from build123d import *

# Parameters (mm, degrees)
ESQUISSE1_W                = 98.15
ESQUISSE1_H                = 27.3
BOSS_EXTRU_1_DEPTH         = 2.7
ESQUISSE2_W                = 10
ESQUISSE2_H                = 2.7
BOSS_EXTRU_2_DEPTH         = 2.7
R_P_TITION_LIN_AIRE1_COUNT = 5
R_P_TITION_LIN_AIRE1_PITCH = 20
ESQUISSE3_W                = 2.7
ESQUISSE3_H                = 6.5
BOSS_EXTRU_3_DEPTH         = 2.7
R_P_TITION_LIN_AIRE2_COUNT = 2
R_P_TITION_LIN_AIRE2_PITCH = 13
ENL_V_MAT_EXTRU_1_DEPTH    = 2.7
CONG_1_R                   = 30
ESQUISSE5_W                = 2.7
ESQUISSE5_H                = 9.15
ENL_V_MAT_EXTRU_2_DEPTH    = 2.7


with BuildPart() as part:
    # Esquisse1 → Boss.-Extru.1 (new body)
    with BuildSketch(Plane.XY):
        with Locations((49.075, -13.65)):
            Rectangle(ESQUISSE1_W, ESQUISSE1_H)
    extrude(amount=BOSS_EXTRU_1_DEPTH)

    # Esquisse2 → Boss.-Extru.2 (add)
    with BuildSketch(Plane.XY):
        with Locations((10, -28.65)):
            Rectangle(ESQUISSE2_W, ESQUISSE2_H)
    boss_extru_2 = extrude(amount=BOSS_EXTRU_2_DEPTH)

    # Répétition linéaire1: Boss.-Extru.2 ×5
    with Locations(*[(i * R_P_TITION_LIN_AIRE1_PITCH, 0, 0) for i in range(1, R_P_TITION_LIN_AIRE1_COUNT)]):
        add(boss_extru_2)

    # Esquisse3 → Boss.-Extru.3 (add)
    with BuildSketch(Plane.XY):
        with Locations((99.5, -6.5)):
            Rectangle(ESQUISSE3_W, ESQUISSE3_H)
    boss_extru_3 = extrude(amount=BOSS_EXTRU_3_DEPTH)

    # Répétition linéaire2: Boss.-Extru.3 ×2
    with Locations(*[(0, -i * R_P_TITION_LIN_AIRE2_PITCH, 0) for i in range(1, R_P_TITION_LIN_AIRE2_COUNT)]):
        add(boss_extru_3)

    # Esquisse4 → Enlèv. mat.-Extru.1 (cut)
    with BuildSketch(Plane.XY):
        Polygon((0, -9), (69.411542732, -9), (85, 0), (0, 0), align=None)
    extrude(amount=ENL_V_MAT_EXTRU_1_DEPTH, mode=Mode.SUBTRACT)

    # Congé1
    cong_1_edges = [part.edges().sort_by_distance(p)[0] for p in [
        (69.411542732, -9, 1.35),
        (85, 0, 1.35),
    ]]
    fillet(cong_1_edges, radius=CONG_1_R)

    # Symétrie1: part across plane


with BuildPart() as part_1:
    add(part.part)
    add(part.part.mirror(Plane(origin=(0, 0, 0), x_dir=(0, 0, 1), z_dir=(1, 0, 0))))

    # Esquisse5 → Enlèv. mat.-Extru.2 (cut)
    with BuildSketch(Plane.XY):
        with Locations((40, -22.725)):
            Rectangle(ESQUISSE5_W, ESQUISSE5_H)
    enl_v_mat_extru_2 = extrude(amount=ENL_V_MAT_EXTRU_2_DEPTH, mode=Mode.SUBTRACT)

    # Symétrie2: Enlèv. mat.-Extru.2 across plane
    add(enl_v_mat_extru_2.mirror(Plane(origin=(0, 0, 0), x_dir=(0, 0, 1), z_dir=(1, 0, 0))), mode=Mode.SUBTRACT)


solid = part_1.part
Could you check a few things on this model? Use its own coordinates, in mm. A direction names the side the tool comes from. Give positions to 0.01 mm unless a question says otherwise; leave off trailing zeros. Write each loop counter-clockwise with the first axis right and the second up, starting at its lowest first coordinate (ties: lowest second). Pieces come first, ordered by that corner, then holes. Notation, with made-up numbers: (-7.5, -15.75) -> (16.5, -15.75) arc R23 ccw to (16.5, -7.75) -> close; hole circle Ø9 at (-36, 39.25). An arc over 180 degrees is marked (long way). Answer as CSV lines item,"result". Start each with the question number.
(1) If we section it at C-C, the plane x = -71.5: Write out the boundary of the cut face in (y, z).
(2) Which directions (+Z, -Z, +X, -X, +Y, -Y) give clear straight access to the entire face, cutting with the end or side of a thin tool? Please do faces 3 (the face through (1, -18, 0)), 4 (the face through (-69.031, -8.006, 1.369)).
(3) If we section it at A-A, the plane y = -20.5: Write out the boundary of the cut face in (x, z), and give its area (3 significant figures).
(4) Please list where these lines run through material, in increasing order: line 1 (X direction, y = -21.5, z = 2.05); line 2 (X direction, y = -26, z = 2); line 3 (Y direction, x = -48, z = 2.2).
(5) If we mould it in two halves opening along X, with no side actions, what happens to faces 1 (the face through (1, -18, 2.7)), 2 (the face through (69.031, -8.006, 1.369))? For each: +X half, -X half, draft (parallel to the pull), parting line (faces both ways), or undercut.
(6) I'm going to push flat-ended pins straight in: pin 1 Ø1.3 at (x, z) = (-99, 2) entering from -Y; pin 2 Ø0.8 at (y, z) = (-29.5, 1.5) entering from +X; pin 3 Ø1.4 at (x, z) = (96.5, 1) entering from -Y. Where does each tip first touch, or does it pass through?
(7) If we section it at B-B, the plane x = 30.5: Write out the boundary of the cut face in (y, z).
Answer list:
1,outline,"(-30, 0) -> (-7.24, 0) -> (-7.24, 2.7) -> (-30, 2.7) -> close"
2,face 3,"-Z, +X, -X, +Y, -Y"
2,face 4,"+Z, -Z, +Y"
3,outline,"(-100.85, 0) -> (-41.35, 0) -> (-41.35, 2.7) -> (-100.85, 2.7) -> close; (-38.65, 0) -> (38.65, 0) -> (38.65, 2.7) -> (-38.65, 2.7) -> close; (41.35, 0) -> (100.85, 0) -> (100.85, 2.7) -> (41.35, 2.7) -> close"
3,area,"530 mm^2"
4,line 1,"-100.85 to -41.35, -38.65 to 38.65, 41.35 to 100.85"
4,line 2,"-98.15 to -41.35, -38.65 to 38.65, 41.35 to 98.15"
4,line 3,"-30 to -9"
5,face 1,"draft"
5,face 2,"undercut"
6,pin 1,"y = -22.75"
6,pin 2,"x = 95"
6,pin 3,"y = -27.3"
7,outline,"(-30, 0) -> (-9, 0) -> (-9, 2.7) -> (-30, 2.7) -> close"
